CAD build for the part. Positions are in the model's coordinates, mm. Give positions to 0.01 mm unless a question says otherwise; leave off trailing zeros. Write each loop counter-clockwise with the first axis right and the second up, starting at its lowest first coordinate (ties: lowest second). Pieces come first, ordered by that corner, then holes. Notation, with made-up numbers: (72.5, -16) - (127.5, -16) arc R14 ccw to (127.5, 5) - close; hole circle Ø2 at (77, 37.25). An arc over 180 degrees is marked (long way). Answer as a JSON object with one key per item and string values.
Autodesk Inventor part; units mm, degrees
ref_plane "Płaszczyzna konstrukcyjna1" through (-38, -4, -10) normal (0, 0, -1) x (0, 1, 0)
ref_plane "YZ Plane" through (0, 0, 0) normal (1, 0, 0) x (0, 1, 0)
ref_plane "XZ Plane" through (0, 0, 0) normal (0, 1, 0) x (-1, 0, 0)
sketch "Szkic1" plane through (0, 0, 0) normal (0, 0, 1) x (1, 0, 0)
  arc A0 (33, -4) -> (27, -4) centre (30, -4) ccw
  arc A1 (-27, -4) -> (-33, -4) centre (-30, -4) ccw
  circle A2 centre (30, -4) radius 3 construction
  circle A3 centre (-30, -4) radius 3 construction
  line L0 (-38, -5) -> (-38, -10)
  line L1 (-38, -10) -> (38, -10)
  line L2 (38, -10) -> (38, -5)
  line L3 (-38, 2) -> (-38, -4) construction
  line L4 (38, -4) -> (38, 2) construction
  arc A4 (27.1716, -5) -> (32.8284, -5) centre (30, -4) ccw
  arc A5 (-32.8284, -5) -> (-27.1716, -5) centre (-30, -4) ccw
  line L5 (-32.8284, -5) -> (-38, -5)
  line L6 (38, -5) -> (32.8284, -5)
  line L7 (27.1716, -5) -> (-27.1716, -5)
  point P0 (0, 0)
  dimension "d1" = 5
ref_plane "Płaszczyzna konstrukcyjna1" through (-38, -4, -10) normal (0, 0, -1) x (0, 1, 0)
extrude "Wyciągnięcie proste1" add sketch "Szkic1" against normal up to surface (10 mm away)
sketch "Szkic2" plane through (-38, -10, 0) normal (0, -1, 0) x (1, 0, 0)
  circle A0 centre (58, -5) radius 1.75
  circle A1 centre (18, -5) radius 1.75
  circle A2 centre (58, -5) radius 2
  circle A3 centre (18, -5) radius 2
  point P0 (38, 0)
  dimension "d4" = 4
  dimension "d5" = 4
extrude "Wyciągnięcie proste2" cut sketch "Szkic2" against normal up to next contours A0 | A1 | A2 | A3
properties part number "6_2xclamp_back"
(1) Probe L1, parallel to Z at x = -20, y = -6.35; L2, parallel to X at y = -8.1, z = -6.5; L3, parallel to X at y = -6.45, z = -8.5. List the from-to ranges inside material, lowest first. Write a range as [from, to].
Answer key:
{"L1": "z = [-10, -7], [-3, 0]", "L2": "x = [-38, -21.32], [-18.68, 18.68], [21.32, 38]", "L3": "x = [-38, -31.73], [-28.27, 28.27], [31.73, 38]"}
(2) Saw through at A-A, the plane x = -20. Give the cut face in (y, z), and give its area (3 significant figures).
Answer key:
{"outline": "(-10, -10) - (-5, -10) - (-5, -7) - (-10, -7) - close; (-10, -3) - (-5, -3) - (-5, 0) - (-10, 0) - close", "area": "30.0 mm²"}
(3) Saw through at B-B, the plane z = -5. Give the cut face in (x, y), and give its area (4 significant figures).
Answer key:
{"outline": "(-38, -10) - (-22, -10) - (-22, -5) - (-27.17, -5) arc R3 cw to (-32.83, -5) - (-38, -5) - close; (-18, -10) - (18, -10) - (18, -5) - (-18, -5) - close; (22, -10) - (38, -10) - (38, -5) - (32.83, -5) arc R3 cw to (27.17, -5) - (22, -5) - close", "area": "323.5 mm²"}
(4) Flat gauge pin, fed straight in: P1, Ø3, axis at x = -20, z = -5, coming from the +Y side. Where does the tip first touch, or does it go through?
Answer key:
{"P1": "passes through"}
(5) Saw through at C-C, the plane y = -8.9. Give the cut face in (x, z), and give its area (3 significant figures).
Answer key:
{"outline": "(-38, -10) - (38, -10) - (38, 0) - (-38, 0) - close; hole circle Ø4 at (-20, -5); hole circle Ø4 at (20, -5)", "area": "735 mm²"}
(6) Saw through at D-D, the plane z = -7.75. Give the cut face in (x, y), and give its area (4 significant figures).
Answer key:
{"outline": "(-38, -10) - (38, -10) - (38, -5) - (32.83, -5) arc R3 cw to (27.17, -5) - (-27.17, -5) arc R3 cw to (-32.83, -5) - (-38, -5) - close", "area": "363.5 mm²"}
(7) Pull direction X, two halves, no side cores. Call faces 1 (the face through (38, -8, -5)), 2 (the face through (-35, -5, -5)), 3 (the face through (-21.6, -7.5, -6.2)), 4 (the face through (-30, -7, -5)): pulls with the +X half, pulls with the -X half, needs draft (parallel to the pull), parting line crosses it, or undercut.
Answer key:
{"face 1": "pulls with the +X half", "face 2": "needs draft", "face 3": "undercut", "face 4": "undercut"}
